from build123d import *

# Parameters (mm, degrees)
F1_DEPTH    = 57.15
F2_T        = 3.683
F2_T3_DEPTH = 64.516
F4_DEPTH    = 25.4
F6_DEPTH    = 6.35
F7_R        = 3.175
F8_DEPTH    = 25.4
F10_DEPTH   = 56.642


# Not quite as in the source:
# - a shell that OpenCascade refuses in one call is made with other operations: the cavity is built on its own and cut out


with BuildPart() as f1:
    # F0 (on Top) → F1 (new body)
    with BuildSketch(Plane.XY):
        with BuildLine():
            ThreePointArc((33.7229068752, -2.2373507569), (35.8958962, -0.5864150612), (38.5611520326, 0))
            Line((38.5611520326, 0), (44.45, 0))
            ThreePointArc((44.45, 0), (48.9401280605, 1.8598719395), (50.8, 6.35))
            Line((50.8, 6.35), (50.8, 38.1))
            ThreePointArc((50.8, 38.1), (48.9401280605, 42.5901280605), (44.45, 44.45))
            Line((44.45, 44.45), (6.35, 44.45))
            ThreePointArc((6.35, 44.45), (1.8598719395, 42.5901280605), (0, 38.1))
            Line((0, 38.1), (0, 13.2369613275))
            ThreePointArc((0, 13.2369613275), (0.138072898, 11.4377303868), (0, 9.6384994461))
            ThreePointArc((0, 9.6384994461), (-2.9389427728, 3.4941811086), (-8.7853716686, 0))
            Line((-8.7853716686, 0), (-17.4601711333, 0))
            ThreePointArc((-17.4601711333, 0), (-22.6964673635, -2.6732403398), (-25.4, -7.893960923))
            Line((-25.4, -7.893960923), (-25.4, -31.2883965671))
            ThreePointArc((-25.4, -31.2883965671), (-29.8218894142, -38.9045945069), (-38.1, -41.91))
            Line((-38.1, -41.91), (-38.1, -73.66))
            Line((-38.1, -73.66), (-28.4519677815, -73.66))
            ThreePointArc((-28.4519677815, -73.66), (-25.7012193429, -73.0332755505), (-23.4934508416, -71.276813552))
            Line((-23.4934508416, -71.276813552), (0, -41.91))
            Line((0, -41.91), (33.7229068752, -2.2373507569))
        make_face()
    extrude(amount=F1_DEPTH)

    # F2: shell of thickness 3.683, made by hand


with BuildPart() as f2_core1:
    # F2_t2: copy of F1
    add(f1.part)

    # the walls: a layer under each face that stays
    f2_faces = [f2_core1.faces().sort_by_distance(p)[0] for p in [
        (35.8958962, -0.5864150612, 28.575),
        (6.35, -14.605, 57.15),
        (-11.7467254208, -56.593406776, 28.575),
        (-25.7012193429, -73.0332755505, 28.575),
        (-33.2759838908, -73.66, 28.575),
        (48.9401280605, 42.5901280605, 28.575),
        (50.8, 22.225, 28.575),
        (48.9401280605, 1.8598719395, 28.575),
        (6.35, -14.605, 0),
        (41.5055760163, 0, 28.575),
        (16.8614534376, -22.0736753784, 28.575),
    ]]
    thicken(f2_faces, amount=-F2_T, mode=Mode.SUBTRACT)

    # F2_s4 → F2_t3 (cut)
    with BuildSketch(Plane.XY.offset(-3.683)):
        Polygon((0.0568212202, -41.9568608842), (-2.8759398252, -39.6092481399), (-2.8416905769, -39.5664365795), (-2.8061821913, -39.524663439), align=None)
    extrude(amount=F2_T3_DEPTH, mode=Mode.SUBTRACT)


with BuildPart() as f1_1:
    add(f1.part)

    # what is left inside the walls is the cavity
    f2_cavity = [f2_core1.part.solids().sort_by_distance(p)[0] for p in [
        (15.160625, 19.021778, 3.71983),
    ]]
    add(f2_cavity, mode=Mode.SUBTRACT)

    # F3 (on face) → F4 (cut)
    with BuildSketch(Plane.YZ.offset(50.8)):
        with BuildLine():
            ThreePointArc((38.1, 7.9580365134), (49.4216390683, 15.7128126042), (53.7828262711, 28.7241964505))
            ThreePointArc((53.7828262711, 28.7241964505), (49.4216390683, 41.7355802968), (38.1, 49.4903563877))
            Line((38.1, 49.4903563877), (38.1, 7.9580365134))
        make_face()
        with BuildLine():
            Line((38.1, 7.9580365134), (38.1, 49.4903563877))
            ThreePointArc((38.1, 49.4903563877), (10.6028262711, 28.7241964505), (38.1, 7.9580365134))
        make_face()
    extrude(amount=-F4_DEPTH, mode=Mode.SUBTRACT)

    # F5 (on face) → F6 (join)
    with BuildSketch(Plane(origin=(0, 0, 0), x_dir=(1, 0, 0), z_dir=(0, 0, -1))):
        with BuildLine():
            Line((33.1074998051, 73.66), (-28.4519677815, 73.66))
            ThreePointArc((-28.4519677815, 73.66), (-25.7012193429, 73.0332755505), (-23.4934508416, 71.276813552))
            Line((-23.4934508416, 71.276813552), (0, 41.91))
            Line((0, 41.91), (33.7229068752, 2.2373507569))
            ThreePointArc((33.7229068752, 2.2373507569), (35.8958962, 0.5864150612), (38.5611520326, 0))
            Line((38.5611520326, 0), (44.45, 0))
            ThreePointArc((44.45, 0), (47.9823010709, -1.0731307441), (50.3207058028, -3.9298112931))
            Line((50.3207058028, -3.9298112931), (45.77730068, 61.8352975433))
            ThreePointArc((45.77730068, 61.8352975433), (41.7727672909, 70.2445645778), (33.1074998051, 73.66))
        make_face()
        with BuildLine():
            Line((-28.4519677815, 73.66), (-38.1, 73.66))
            Line((-38.1, 73.66), (-38.1, 41.91))
            ThreePointArc((-38.1, 41.91), (-29.7548118209, 38.9847975987), (-25.4, 31.2883965671))
            Line((-25.4, 31.2883965671), (-25.4, 7.893960923))
            ThreePointArc((-25.4, 7.893960923), (-22.5976268538, 2.7726551632), (-17.4601711333, 0))
            Line((-17.4601711333, 0), (-8.7853716686, 0))
            ThreePointArc((-8.7853716686, 0), (-1.8289491462, -4.9169285395), (0, -13.2369613275))
            Line((0, -13.2369613275), (0, -38.1))
            ThreePointArc((0, -38.1), (1.8598719395, -42.5901280605), (6.35, -44.45))
            Line((6.35, -44.45), (44.45, -44.45))
            ThreePointArc((44.45, -44.45), (48.9401280605, -42.5901280605), (50.8, -38.1))
            Line((50.8, -38.1), (50.8, -10.8675230294))
            Line((50.8, -10.8675230294), (50.3207058028, -3.9298112931))
            ThreePointArc((50.3207058028, -3.9298112931), (47.9823010709, -1.0731307441), (44.45, 0))
            Line((44.45, 0), (38.5611520326, 0))
            ThreePointArc((38.5611520326, 0), (35.8958962, 0.5864150612), (33.7229068752, 2.2373507569))
            Line((33.7229068752, 2.2373507569), (0, 41.91))
            Line((0, 41.91), (-23.4934508416, 71.276813552))
            ThreePointArc((-23.4934508416, 71.276813552), (-25.7012193429, 73.0332755505), (-28.4519677815, 73.66))
        make_face()
    extrude(amount=F6_DEPTH)

    # F7 (on face) → F8 (cut)
    with BuildSketch(Plane.XY):
        with Locations((0, -63.8569965959)):
            Circle(F7_R)
        with Locations((33.1074998051, -60.96)):
            Circle(F7_R)
        with Locations((34.9028557539, -18.2985700667)):
            Circle(F7_R)
    extrude(amount=-F8_DEPTH, mode=Mode.SUBTRACT)

    # F9 (on face) → F10 (join)
    with BuildSketch(Plane.XY.offset(57.15)):
        with BuildLine():
            Line((-9.8974186925, -28.5147787669), (-13.1322266534, -52.4904169142))
            Line((-13.1322266534, -52.4904169142), (23.2126582414, -8.8060172275))
            Line((23.2126582414, -8.8060172275), (-1.8316966669, -18.3445471934))
            ThreePointArc((-1.8316966669, -18.3445471934), (-7.2620315182, -22.3213661397), (-9.8974186925, -28.5147787669))
        make_face()
        with BuildLine():
            Line((-28.4519677815, -65.1904169142), (-28.4519677815, -67.31))
            Line((-28.4519677815, -67.31), (-27.7152992785, -69.8403045535))
            Line((-27.7152992785, -69.8403045535), (-13.1322266534, -52.4904169142))
            Line((-13.1322266534, -52.4904169142), (-15.7519677815, -52.4904169142))
            ThreePointArc((-15.7519677815, -52.4904169142), (-24.7322239026, -56.2101607932), (-28.4519677815, -65.1904169142))
        make_face()
    extrude(amount=-F10_DEPTH)


solid = f1_1.part
Work out the finished part from the listing and answer in its coordinate system (mm). A direction names the side the tool comes from. Give positions to 0.01 mm unless a question says otherwise; leave off trailing zeros. Loops run counter-clockwise (first coordinate to the right, second up) from the corner with the lowest first, then second, coordinate; pieces in that order, holes last. Notation, with made-up numbers: M 25,55.5 L 45,55.5 A20 ccw 45,90.5 Z; hole C 48.25,32.5 d3. An arc over 180 degrees is marked long. Use CSV: the item, a comma, the result in double quotes.
1) Find section B-B on z = 24.5. Write down the section's boundary in (x, y).
Answer:
outline,"M -38.1,-73.66 L -28.45,-73.66 A6.35 ccw -23.49,-71.28 L 0,-41.91 L 33.72,-2.24 A6.35 cw 38.56,0 L 44.45,0 A6.35 ccw 50.8,6.35 L 50.8,11.02 L 47.12,11.02 L 47.12,6.35 A2.67 cw 44.45,3.68 L 38.56,3.68 A10.03 ccw 30.92,0.15 L 18.93,-13.96 L 23.21,-8.81 L -1.83,-18.34 A12.7 ccw -9.9,-28.51 L -13.12,-52.42 L -13.18,-52.49 L -15.75,-52.49 A12.7 ccw -28.45,-65.19 L -28.45,-67.31 L -27.72,-69.84 L -14.14,-53.69 L -26.37,-68.98 A2.67 cw -28.45,-69.98 L -38.1,-69.98 Z"
2) Find section C-C on x = -32. Write down the section's boundary in (y, z), plus the area to 3 significant figures.
Answer:
outline,"M -73.66,-6.35 L -40.48,-6.35 L -40.48,0 L -40.38,0 L -40.38,3.68 L -69.98,3.68 L -69.98,53.47 L -40.38,53.47 L -40.38,57.15 L -73.66,57.15 Z"
area,"639 mm^2"
3) Which of the six approach directions +Z, -Z, +X, -X, +Y, -Y give full straight-line access (tool end or side, diameter ignored) to faces 5 (the flat face through (-33, -69.977, 28)), 6 (the cylindrical face through (48.99, 42.54, 51.75)), 7 (the flat face through (-25.4, -19, 55))?
Answer:
face 5,"-X, +Y"
face 6,"+Z, -Z, +X, +Y"
face 7,"+Z, -Z, -X, +Y"
4) Consider L1, parallel to Z at x = -19, y = -16; L2, parallel to X at y = -66, z = 29; L3, parallel to Y at x = 44, z = 7. Determine where each line is inside the solid, lowest interval first.
Answer:
L1,"-6.35 to 3.68, 53.47 to 57.15"
L2,"-28.45 to -24.49, -23.99 to -19.27"
L3,"0 to 3.68"
5) Determine the mould class of faces 1 (the flat face through (50.8, 12, 19)), 2 (the flat face through (48.324, -24.975, -3.131)), 3 (the cylindrical face through (46.315, 4.444, 28.227)), 4 (the flat face through (-20.34, -61.44, 28.23)) for opening direction Y: released by +Y, released by -Y, zero draft, split by the parting line, or undercut.
Answer:
face 1,"zero draft"
face 2,"released by -Y"
face 3,"undercut"
face 4,"undercut"
6) Find section A-A on y = 25.5. Write down the section's boundary in (x, z), plus the area to 3 significant figures.
Answer:
outline,"M 0,-6.35 L 50.8,-6.35 L 50.8,8.2 L 47.12,8.2 L 47.12,3.68 L 0,3.68 Z; M 0,53.47 L 47.12,53.47 L 47.12,49.25 L 50.8,49.25 L 50.8,57.15 L 0,57.15 Z"
area,"729 mm^2"
7) Given P1, Ø1.5, axis at x = 38, z = 50.5, coming from the -Y side; P2, Ø1.1, axis at y = -16, z = 55.5, coming from the -X side; P3, Ø12, axis at x = -1.5, z = 3.5, coming from the -Y side; P4, Ø1.1, axis at y = -66.5, z = 35, coming from the -X side, each flat-ended and moving along its own axis, determine where each tip first touches the part or whether it passes through.
Answer:
P1,"y = -0.14"
P2,"x = -25.4"
P3,"y = -73.66"
P4,"x = -28.45"
8) Find section D-D on y = -36.5. Write down the section's boundary in (x, z).
Answer:
outline,"M -27.6,0 L -27.49,0 L -27.49,-6.35 L 47.53,-6.35 L 47.53,0 L 4.6,0 L 4.6,57.15 L -27.6,57.15 L -27.6,53.47 L -10.97,53.47 L -10.97,3.68 L -27.6,3.68 Z"
